Could you check a few things on this drawing? It's one solid part, dimensions in mm from its lowest x, y, z. A direction names the side the tool comes from. Give positions to 0.01 mm unless a question says otherwise; leave off trailing zeros. Write each loop counter-clockwise with the first axis right and the second up, starting at its lowest first coordinate (ties: lowest second). Pieces come first, ordered by that corner, then holes. Notation, with made-up numbers: M 71.25,-30.5 L 115.25,-30.5 A5 ccw 115.25,-23.5 Z; hole C 2,-22.5 d3. An arc over 180 degrees is marked long. Write each question's results on one line, items separated by ' | '.
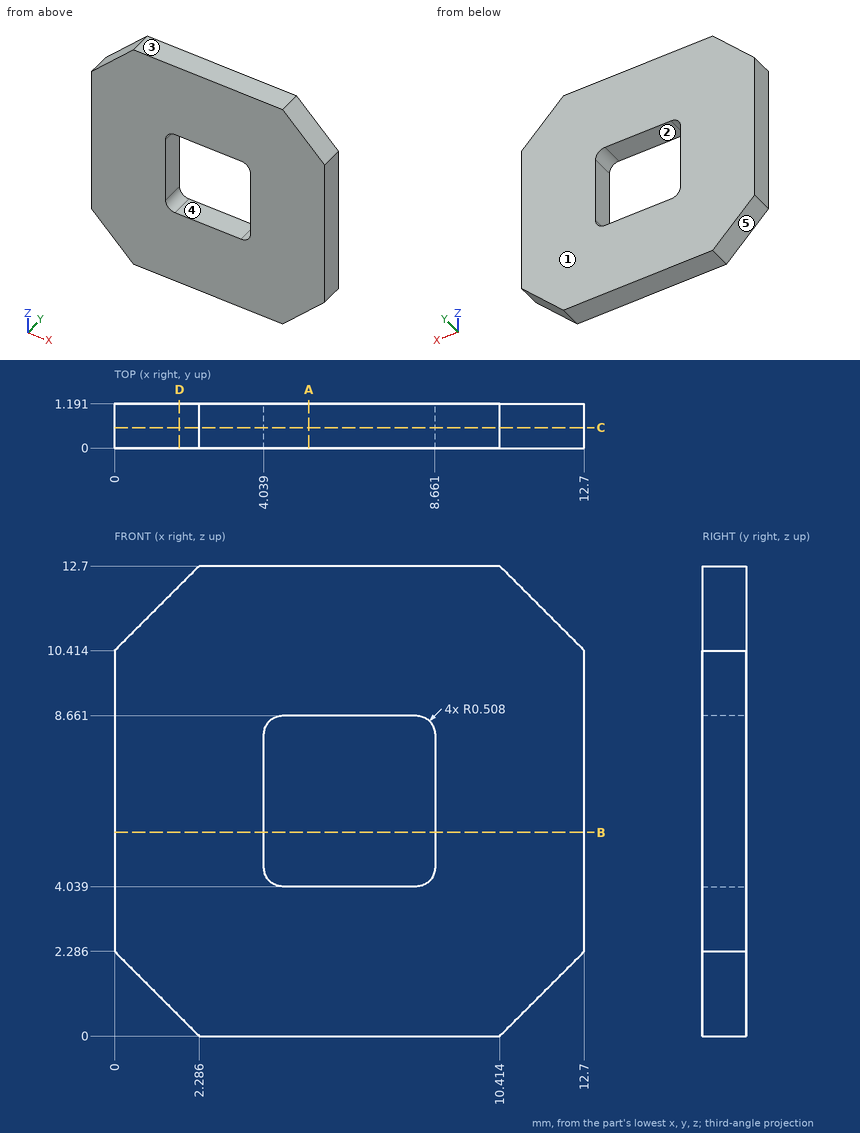
Item 1: If I drill on line 1 (X direction, y = 0.15, z = 6.5); line 2 (X direction, y = 0.65, z = 8.5) (1 decimal), over which ranges is the centre line in solid material (lowest first)? Write a range as from..to.
Geometry says:
line 1: x = 0..4.04, 8.66..12.7 | line 2: x = 0..4.2, 8.5..12.7
Item 2: For the marked faces 1 and 2, which set-ups out of +Z, -Z, +X, -X, +Y, -Y let a thin tool reach every point of the face, with its end or its side?
Geometry says:
face 1: +Z, -Z, +X, -X, +Y | face 2: +Y, -Y
Item 3: Thinking about a two-plate mould opening in X: for the marked faces 3, 4 and 5, which applies, +X half, -X half, draft (parallel to the pull), parting line (faces both ways), or undercut?
Geometry says:
face 3: draft | face 4: undercut | face 5: -X half
Item 4: I want a section at C-C, the plane y = 0.55. Please give me the cut outline in (x, z), and give its area (3 significant figures).
Geometry says:
outline: M 0,2.29 L 2.29,0 L 10.41,0 L 12.7,2.29 L 12.7,10.41 L 10.41,12.7 L 2.29,12.7 L 0,10.41 Z; hole M 4.04,4.55 A0.51 ccw 4.55,4.04 L 8.15,4.04 A0.51 ccw 8.66,4.55 L 8.66,8.15 A0.51 ccw 8.15,8.66 L 4.55,8.66 A0.51 ccw 4.04,8.15 Z | area: 130 mm2
Item 5: I want a section at D-D, the plane x = 1.75. Please give me the cut outline in (y, z).
Geometry says:
outline: M 0,0.54 L 1.19,0.54 L 1.19,12.16 L 0,12.16 Z
Item 6: I want a section at B-B, the plane z = 5.5. Please give me the cut outline in (x, y).
Geometry says:
outline: M 0,0 L 4.04,0 L 4.04,1.19 L 0,1.19 Z; M 8.66,0 L 12.7,0 L 12.7,1.19 L 8.66,1.19 Z
Item 7: I want a section at A-A, the plane x = 5.25. Please give me the cut outline in (y, z).
Geometry says:
outline: M 0,0 L 1.19,0 L 1.19,4.04 L 0,4.04 Z; M 0,8.66 L 1.19,8.66 L 1.19,12.7 L 0,12.7 Z
